Build history of the part. All positions in model axes, mm. A direction names the side the tool comes from. Give positions to 0.01 mm unless a question says otherwise; leave off trailing zeros. Order: outer loops, then holes, each group sorted by start corner. A loop starts at its lowest first (then second) coordinate and runs counter-clockwise, first axis right, second up. Notation, with made-up numbers: (62.5, -22) -> (68.5, -22) arc R19 ccw to (68.5, 14) -> close; hole circle Ø8 at (8.5, -39.5). An arc over 180 degrees is marked (long way). Write item = value, one per line. Start each with the question number.
from build123d import *

# Parameters (mm, degrees)
SKETCH1_R           = 15
SKETCH1_R_2         = 15.000000000000004
BOSS_EXTRUDE1_DEPTH = 50
BOSS_EXTRUDE2_DEPTH = 105
SKETCH4_W           = 80
SKETCH4_H           = 45.000000000000014
BOSS_EXTRUDE4_DEPTH = 8
CUT_EXTRUDE1_DEPTH  = 8
CUT_EXTRUDE2_DEPTH  = 242.98398707352516
FILLET1_R           = 20


with BuildPart() as part:
    # Sketch1 → Boss-Extrude1 (new, symmetric)
    with BuildSketch(Plane(origin=(0, 0, 0), x_dir=(1, 0, 0), z_dir=(0, 1, 0))):
        with BuildLine():
            ThreePointArc((-29.999999999999954, -145), (-35.85786437626902, -159.14213562373092), (-49.99999999999994, -164.99999999999997))
            Line((-49.99999999999994, -164.99999999999997), (49.99999999999994, -164.99999999999994))
            ThreePointArc((49.99999999999994, -164.99999999999997), (35.85786437626901, -159.14213562373092), (29.99999999999996, -145))
            Line((29.99999999999995, -145), (29.99999999999995, -114.78240283248999))
            ThreePointArc((29.999999999999947, -114.78240283248999), (30.981812182919555, -111.80680765393048), (33.541666666666615, -109.99980271446958))
            ThreePointArc((33.54166666666663, -109.99980271446958), (36.78699280171476, -108.95740984718105), (40.00000000000003, -107.81929326423909))
            Line((40.00000000000003, -107.81929326423909), (40.000000000000014, 107.81929326423909))
            ThreePointArc((40.000000000000014, 107.81929326423909), (1.243e-14, 114.99999999999996), (-39.99999999999999, 107.81929326423912))
            Line((-39.999999999999986, 107.81929326423912), (-39.99999999999996, -107.81929326423912))
            ThreePointArc((-39.99999999999996, -107.81929326423912), (-36.78699280171471, -108.95740984718105), (-33.54166666666661, -109.99980271446955))
            ThreePointArc((-33.541666666666615, -109.99980271446958), (-30.981812182919555, -111.80680765393048), (-29.999999999999947, -114.78240283248999))
            Line((-29.99999999999995, -114.78240283248999), (-29.99999999999995, -145))
        make_face()
        with Locations(Location((3.698e-14, -75, 0), (0, 0, 270))):
            Circle(SKETCH1_R, mode=Mode.SUBTRACT)
        with Locations(Location((0, 75, 0), (0, 0, 270))):
            Circle(SKETCH1_R_2, mode=Mode.SUBTRACT)
    extrude(amount=BOSS_EXTRUDE1_DEPTH, both=True)

    # Sketch1_3 → Boss-Extrude2 (add, symmetric)
    with BuildSketch(Plane(origin=(0, 0, 0), x_dir=(1, 0, 0), z_dir=(0, 1, 0))):
        Polygon((-57.49999999999996, -194.99999999999997), (57.50000000000005, -194.99999999999994), (57.50000000000005, -164.99999999999994), (-57.49999999999996, -164.99999999999997), align=None)
    extrude(amount=BOSS_EXTRUDE2_DEPTH, both=True)

    # Sketch4 → Boss-Extrude4 (add)
    with BuildSketch(Plane(origin=(0, 50, 0), x_dir=(1, 0, 0), z_dir=(0, 1, 0))):
        Rectangle(SKETCH4_W, SKETCH4_H)
    extrude(amount=BOSS_EXTRUDE4_DEPTH)

    # Sketch5 → Cut-Extrude1 (cut)
    with BuildSketch(Plane.XZ.offset(50)):
        Polygon((-39.999999999999986, 22.500000000000007), (40.000000000000014, 22.49999999999998), (40.00000000000002, -22.500000000000007), (-39.999999999999986, -22.500000000000007), align=None)
    extrude(amount=-CUT_EXTRUDE1_DEPTH, mode=Mode.SUBTRACT)

    # Sketch6 → Cut-Extrude2 (cut, through all)
    with BuildSketch(Plane.ZY.offset(39.99999999999997)):
        with BuildLine():
            Line((-32.5, 0), (-32.5, -50))
            Line((-32.5, -50), (32.5, -50))
            Line((32.5, -50), (32.5, 0))
            ThreePointArc((32.5, 0), (1.99e-15, 32.5), (-32.5, 0))
        make_face()
    extrude(amount=-CUT_EXTRUDE2_DEPTH, mode=Mode.SUBTRACT)

    # Fillet1
    fillet1_edges = [part.edges().sort_by_distance(p)[0] for p in [
        (0, 50, 164.99999999999997),
        (0, -50, 164.99999999999997),
    ]]
    fillet(fillet1_edges, radius=FILLET1_R)


solid = part.part
(1) Cut at A-A, the plane y = -4. Give the cut face in (x, z), plus the area to 3 significant figures.
(2) 3-axis set-ups, long thin cutter, end or side, ignore diameter. For faces 5 (the face through (30, 1, 130)), 6 (the face through (-30, 1, 130)), 7 (the face through (-50.3, 24.8, 165)): which of +Z, -Z, +X, -X, +Y, -Y reach the whole face in a straight line?
(3) Wall check: line 1 (X direction, y = 24, z = 75); line 2 (Z direction, x = -1, y = 10); line 3 (Z direction, x = -50, y = 93.5). Give the ranges that are in metal, low to high. Write a range as [from, to].
(4) Cut at C-C, the plane x = 0. Give the cut face in (y, z).
(5) Cut at B-B, the plane z = 84. Give the cut face in (x, y), plus the area to 3 significant figures.
(6) Mould opens along Z. For faces 1 (the face through (-1, -25, -32.5)), 2 (the face through (-1, -50, -56)), 3 (the face through (-1, 1, 195)), 4 (the face through (0.7, -58.7, 161.5)) say: released by +Z, released by -Z, zero draft, split by the parting line, or undercut.
(7) Flat gauge pins, fed straight in: P1, Ø4, axis at y = 44.5, z = 35.5, coming from the -X side; P2, Ø2.5, axis at x = 7.5, y = 55.5, coming from the -Z side; P3, Ø10, axis at x = 39, y = 66.5, coming from the -Z side. Where does each tip first touch, or does it go through?
(8) Cut at D-D, the plane y = 24. Give the cut face in (x, z).
Results:
q1.outline = (-57.5, 165) -> (-50, 165) arc R20 cw to (-30, 145) -> (-30, 114.78) arc R5 cw to (-33.54, 110) arc R115 ccw to (-40, 107.82) -> (-40, 32.5) -> (40, 32.5) -> (40, 107.82) arc R115 ccw to (33.54, 110) arc R5 cw to (30, 114.78) -> (30, 145) arc R20 cw to (50, 165) -> (57.5, 165) -> (57.5, 195) -> (-57.5, 195) -> close; (-40, -107.82) arc R115 ccw to (40, -107.82) -> (40, -32.5) -> (-40, -32.5) -> close; hole circle Ø30 at (0, -75); hole circle Ø30 at (0, 75)
q1.area = 18,100 mm2
q2.face_5 = +X, +Y, -Y
q2.face_6 = -X, +Y, -Y
q2.face_7 = -Z
q3.line_1 = [-40, -15], [15, 40]
q3.line_2 = [-115, -89.97], [-60.03, -30.92], [30.92, 60.03], [89.97, 195]
q3.line_3 = [165, 195]
q4.outline = (-105, 165) -> (-70, 165) arc R20 cw to (-50, 145) -> (-50, 90) -> (50, 90) -> (50, 145) arc R20 cw to (70, 165) -> (105, 165) -> (105, 195) -> (-105, 195) -> close; (-50, -115) -> (50, -115) -> (50, -90) -> (-50, -90) -> close; (-50, -60) -> (50, -60) -> (50, -22.5) -> (58, -22.5) -> (58, 22.5) -> (50, 22.5) -> (50, 60) -> (-50, 60) -> (-50, 32.5) -> (0, 32.5) arc R32.5 cw to (0, -32.5) -> (-50, -32.5) -> close
q5.outline = (-40, -50) -> (-12, -50) -> (-12, 50) -> (-40, 50) -> close; (12, -50) -> (40, -50) -> (40, 50) -> (12, 50) -> close
q5.area = 5,600 mm2
q6.face_1 = undercut
q6.face_2 = zero draft
q6.face_3 = released by +Z
q6.face_4 = released by -Z
q7.P1 = -40
q7.P2 = -22.5
q7.P3 = 163.1
q8.outline = (-57.5, 165) -> (-50, 165) arc R20 cw to (-30, 145) -> (-30, 114.78) arc R5 cw to (-33.54, 110) arc R115 ccw to (-40, 107.82) -> (-40, 21.91) -> (40, 21.91) -> (40, 107.82) arc R115 ccw to (33.54, 110) arc R5 cw to (30, 114.78) -> (30, 145) arc R20 cw to (50, 165) -> (57.5, 165) -> (57.5, 195) -> (-57.5, 195) -> close; (-40, -107.82) arc R115 ccw to (40, -107.82) -> (40, -21.91) -> (-40, -21.91) -> close; hole circle Ø30 at (0, -75); hole circle Ø30 at (0, 75)
